Could you check a few things on this model? Use its own coordinates, in mm. Give positions to 0.01 mm unless a question says otherwise; leave off trailing zeros. Loops run counter-clockwise (first coordinate to the right, second up) from the corner with the lowest first, then second, coordinate; pieces in that order, holes last. Notation, with made-up numbers: (-24, 88.25) - (-15, 88.25) arc R8 ccw to (-15, 97.25) - close; hole circle Ø11 at (-5.75, -37). An arc over 180 degrees is marked (long way). One line per item, written item: value. Start each with the question number.
Q1. I want a section at C-C (x = 28.5). Please give me the cut outline in (y, z), then the cut area to 3 significant figures.
Q2. I'm going to push a flat-ended pin straight in: P1, Ø7.5, axis at x = 41.529, y = 25.4, coming from the +Z side. Where does the tip first touch, or does it pass through?
Q3. If I drill on line 1 (Y direction, x = 40.5, z = 1.55); line 2 (Y direction, x = 23.5, z = 1.35); line 3 (X direction, y = 23, z = 0.65) (3 decimals), over which ranges is the centre line in solid material (lowest first)? Write a range as from..to.
Q4. I want a section at D-D (x = 15). Please give me the cut outline in (y, z).
Q5. If we mould it in two halves opening along X, with no side actions, what happens to faces 1 (the face through (26.8, 30.085, 0.783)), 2 (the face through (23, 0, 1)), 3 (the face through (47.625, 13, 1))? For each: released by +X, released by -X, zero draft, split by the parting line, or undercut.
Q6. I want a section at B-B (z = 1.1). Count the separate pieces of the cut face and the enclosed holes in it, then the cut area to 3 significant figures.
Q7. I want a section at A-A (x = 21). Please give me the cut outline in (y, z).
```python
from build123d import *

# Parameters (mm, degrees)
SKETCH1_R           = 5.55625
SKETCH1_R_2         = 2.921
BOSS_EXTRUDE1_DEPTH = 1.5875


with BuildPart() as part:
    # Sketch1 → Boss-Extrude1 (new body)
    with BuildSketch(Plane.XY):
        with BuildLine():
            Line((0, 0), (47.625, 0))
            Line((47.625, 0), (47.625, 25.4))
            ThreePointArc((47.625, 25.4), (43.704494442, 31.094597434), (36.985748053, 29.464489851))
            ThreePointArc((36.985748053, 29.464489851), (35.819445625, 29.06042219), (34.860756534, 29.83788425))
            ThreePointArc((34.860756534, 29.83788425), (23.8125, 37.30625), (12.764243466, 29.83788425))
            ThreePointArc((12.764243466, 29.83788425), (11.805554375, 29.06042219), (10.639251947, 29.464489851))
            ThreePointArc((10.639251947, 29.464489851), (3.920505558, 31.094597434), (0, 25.4))
            Line((0, 25.4), (0, 0))
        make_face()
        with Locations((23.8125, 25.4)):
            Circle(SKETCH1_R, mode=Mode.SUBTRACT)
        with Locations((6.096, 25.4)):
            Circle(SKETCH1_R_2, mode=Mode.SUBTRACT)
        with Locations((41.529, 25.4)):
            Circle(SKETCH1_R_2, mode=Mode.SUBTRACT)
    extrude(amount=BOSS_EXTRUDE1_DEPTH)


solid = part.part
```
Worked answers:
1. outline: (0, 0) - (22.42, 0) - (22.42, 1.59) - (0, 1.59) - close; (28.38, 0) - (36.34, 0) - (36.34, 1.59) - (28.38, 1.59) - close
1. area: 48.2 mm²
2. P1: stops at z = 1.59
3. line 1: y = 0..22.67, 28.13..31.41
3. line 2: y = 0..19.85, 30.95..37.3
3. line 3: x = 0..4.431, 7.761..18.801, 28.824..39.864, 43.194..47.625
4. outline: (0, 0) - (33.41, 0) - (33.41, 1.59) - (0, 1.59) - close
5. face 1: undercut
5. face 2: zero draft
5. face 3: released by +X
6. separate pieces: 1
6. enclosed holes: 3
6. area: 1,400 mm²
7. outline: (0, 0) - (20.61, 0) - (20.61, 1.59) - (0, 1.59) - close; (30.19, 0) - (36.97, 0) - (36.97, 1.59) - (30.19, 1.59) - close
